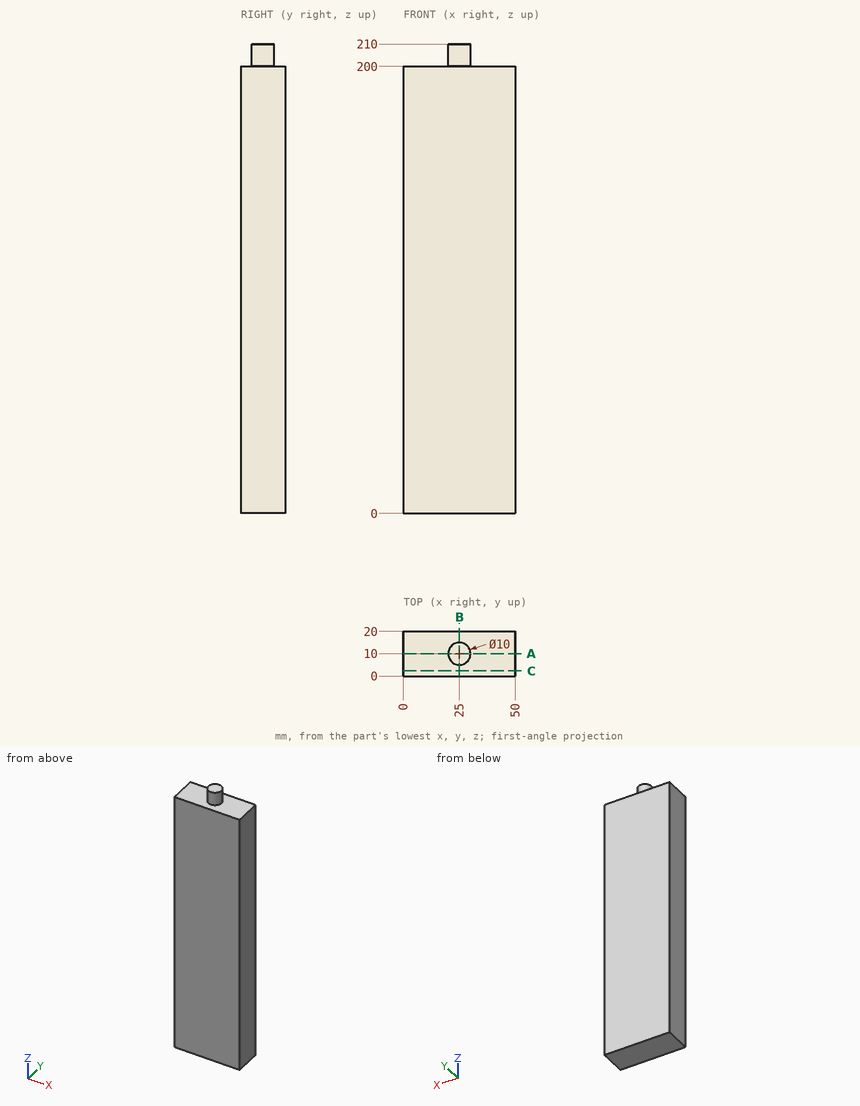
Source: three-view drawing plus pictorial views. Frame: mm from the lowest corner of the part. Round coordinates to 2 decimals unless told otherwise and drop trailing zeros. Loops run counter-clockwise (first coordinate to the right, second up) from the corner with the lowest first, then second, coordinate; pieces in that order, holes last. Notation, with made-up numbers: M 5,67 L 55,67 A20 ccw 55,97 Z; hole C -28.5,69 d2. An arc over 180 degrees is marked long. Answer as CSV lines item,"result". Start each with the question number.
(1) Section A-A, the plane y = 10. Output: boundary loops of the cut face in (x, z).
(2) Line query: line 1 (Z direction, x = 16, y = 19.25). Output: solid intervals per line, ascending. Write a range as [from, to].
(3) Section B-B, the plane x = 25. Output: boundary loops of the cut face in (y, z).
(4) First-contact query: pin 1 (6 mm diameter, centred on x = 6.5, y = 14, fed in from +Z). Flat tip, straight axial feed; report the tip coordinate or a pass-through.
(5) Section C-C, the plane y = 2.25. Output: boundary loops of the cut face in (x, z), plus the area to 3 significant figures.
Values found:
1,outline,"M 0,0 L 50,0 L 50,200 L 30,200 L 30,210 L 20,210 L 20,200 L 0,200 Z"
2,line 1,"z = [0, 200]"
3,outline,"M 0,0 L 20,0 L 20,200 L 15,200 L 15,210 L 5,210 L 5,200 L 0,200 Z"
4,pin 1,"stops at z = 200"
5,outline,"M 0,0 L 50,0 L 50,200 L 0,200 Z"
5,area,"10,000 mm²"
